```python
from build123d import *

# Parameters (mm, degrees)
SKETCH1_R           = 50.5
SKETCH1_R_2         = 36
BOSS_EXTRUDE1_DEPTH = 16
SKETCH2_R           = 2.5
CUT_EXTRUDE1_DEPTH  = 74.188113789
SKETCH3_R           = 4.5
CUT_EXTRUDE2_DEPTH  = 13
FILLET1_R           = 7


with BuildPart() as part:
    # Sketch1 → Boss-Extrude1 (new body)
    with BuildSketch(Plane(origin=(0, 0, 0), x_dir=(1, 0, 0), z_dir=(0, 1, 0))):
        with Locations(Location((0, 0, 0), (0, 0, 270))):
            Circle(SKETCH1_R)
        with Locations(Location((0, 0, 0), (0, 0, 270))):
            Circle(SKETCH1_R_2, mode=Mode.SUBTRACT)
    extrude(amount=BOSS_EXTRUDE1_DEPTH)

    # Sketch2 → Cut-Extrude1 (cut, through all)
    with BuildSketch(Plane(origin=(0, 16, 0), x_dir=(1, 0, 0), z_dir=(0, 1, 0))):
        with Locations(Location((0, 43.5, 0), (0, 0, 270))):
            Circle(SKETCH2_R)
        with Locations(Location((37.672105065, 21.75, 0), (0, 0, 270))):
            Circle(SKETCH2_R)
        with Locations(Location((37.672105065, -21.75, 0), (0, 0, 270))):
            Circle(SKETCH2_R)
        with Locations(Location((0, -43.5, 0), (0, 0, 270))):
            Circle(SKETCH2_R)
        with Locations(Location((-37.672105065, -21.75, 0), (0, 0, 270))):
            Circle(SKETCH2_R)
        with Locations(Location((-37.672105065, 21.75, 0), (0, 0, 270))):
            Circle(SKETCH2_R)
    extrude(amount=-CUT_EXTRUDE1_DEPTH, mode=Mode.SUBTRACT)

    # Sketch3 → Cut-Extrude2 (cut)
    with BuildSketch(Plane.XZ):
        with BuildLine():
            Line((0, 0), (8.769232972, 49.732791527))
            ThreePointArc((8.769232972, 49.732791527), (43.734282891, 25.25), (47.45447735, -17.272017238))
            Line((47.45447735, -17.272017238), (0, 0))
        make_face()
        with Locations(Location((37.672105065, 21.75, 0), (0, 0, 270))):
            Circle(SKETCH3_R, mode=Mode.SUBTRACT)
    extrude(amount=-CUT_EXTRUDE2_DEPTH, mode=Mode.SUBTRACT)

    # Fillet1
    fillet1_edges = [part.edges().sort_by_distance(p)[0] for p in [
        (6.251334396, 6.5, 35.453079108),
        (33.828934348, 6.5, -12.31272516),
        (47.45447735, 6.5, -17.272017238),
        (8.769232972, 6.5, 49.732791527),
    ]]
    fillet(fillet1_edges, radius=FILLET1_R)


solid = part.part
```
Here's how the part is built. I have some questions about the finished solid (model axes, mm). A direction names the side the tool comes from. Round coordinates to 2 decimals unless told otherwise and drop trailing zeros. Order: outer loops, then holes, each group sorted by start corner. A loop starts at its lowest first (then second) coordinate and runs counter-clockwise, first axis right, second up. Notation, with made-up numbers: (-30.75, 27) -> (-11.75, 27) arc R21 cw to (-11.75, 47) -> close; hole circle Ø5 at (17, 45.25). An arc over 180 degrees is marked (long way). Use a Markdown table: item, result. Add a question column.
(1) Suppose I cut it at B-B, the plane y = 10.75. Please give me the cut outline in (x, z), and give its area (3 significant figures).
(2) Suppose I cut it at C-C, the plane x = -8. Please give me the cut outline in (y, z).
(3) For pin 1 Ø3 at (x, y) = (-18, 5.5) entering from -Z; pin 2 Ø4 at (x, z) = (-37.67, -21.75) entering from -Y; pin 3 Ø1.5 at (y, z) = (7.5, -22.5) entering from +X; pin 4 Ø2 at (x, y) = (15.5, 5) entering from +Z, each with a flat end and sliding along its axis, tell me the tip position at first contact or that it passes through.
(4) Suppose I cut it at D-D, the plane z = 43.5. Please give me the cut outline in (x, y), and give its area (3 significant figures).
(5) For faces 1 (the face through (35.11, 6.41, -14.5)), 2 (the face through (44.541, 6.591, -18.905)), 3 (the face through (-34.4, 0, -11.5)), which set-ups out of +Z, -Z, +X, -X, +Y, -Y let a thin tool reach every point of the face, with its end or its side?
(6) Suppose I cut it at A-A, the plane z = 0. Please give me the cut outline in (x, y), and give its area (4 significant figures).
(7) I need wall thicknesses on line 1 along X through (y, z) = (6, -21.75); line 2 along X through (y, z) = (3.5, 21.75); line 3 along Z through (x, y) = (-37, 6.5). Which ranges of each line are inside material? Lowest first, please.
(8) If we mould it in two halves opening along X, with no side actions, what happens to faces 4 (the face through (5.898, 6.591, 48.026)), 5 (the face through (-49.3, 7.89, -10.95)), 6 (the face through (15, 16, 33)), 7 (the face through (42.134, 6.409, 22.336))? For each: released by +X, released by -X, zero draft, split by the parting line, or undercut.
Verdict:
| question | item | result |
|---|---|---|
| 1 | outline | (0.4, 36) arc R7 ccw to (7.37, 41.78) -> (7.46, 42.28) arc R7 ccw to (0.65, 50.5) arc R50.5 ccw (long way) to (44.06, -24.68) arc R7 ccw to (40.34, -14.68) -> (39.87, -14.51) arc R7 ccw to (31.37, -17.66) arc R36 cw (long way) to start; circle Ø9 at (37.67, 21.75); hole circle Ø5 at (-37.67, -21.75); hole circle Ø5 at (-37.67, 21.75); hole circle Ø5 at (0, -43.5); hole circle Ø5 at (0, 43.5); hole circle Ø5 at (37.67, -21.75); hole circle Ø5 at (37.67, 21.75) |
| 1 | area | 2,750 mm2 |
| 2 | outline | (0, -49.86) -> (16, -49.86) -> (16, -35.1) -> (0, -35.1) -> close; (0, 35.1) -> (16, 35.1) -> (16, 49.86) -> (0, 49.86) -> close |
| 3 | pin 1 | z = -47.73 |
| 3 | pin 2 | through |
| 3 | pin 3 | x = 44.93 |
| 3 | pin 4 | z = -32 |
| 4 | outline | (-25.65, 0) -> (-2.5, 0) -> (-2.5, 16) -> (-25.65, 16) -> close; (2.5, 0) -> (7.56, 0) -> (7.56, 13) -> (25.65, 13) -> (25.65, 16) -> (2.5, 16) -> close |
| 4 | area | 506 mm2 |
| 5 | face 1 | -Y |
| 5 | face 2 | +X, -Y |
| 5 | face 3 | +Z, -Z, +X, -X, -Y |
| 6 | outline | (-50.5, 0) -> (-36, 0) -> (-36, 16) -> (-50.5, 16) -> close; (36, 13) -> (50.5, 13) -> (50.5, 16) -> (36, 16) -> close |
| 6 | area | 275.5 mm2 |
| 7 | line 1 | -45.58 to -40.17, -35.17 to -28.69, 28.69 to 35.17, 40.17 to 44.93 |
| 7 | line 2 | -45.58 to -40.17, -35.17 to -28.69, 33.17 to 35.17, 40.17 to 42.17 |
| 7 | line 3 | -34.37 to -24.16, -19.34 to 19.34, 24.16 to 34.37 |
| 8 | face 4 | released by +X |
| 8 | face 5 | split by the parting line |
| 8 | face 6 | zero draft |
| 8 | face 7 | undercut |
